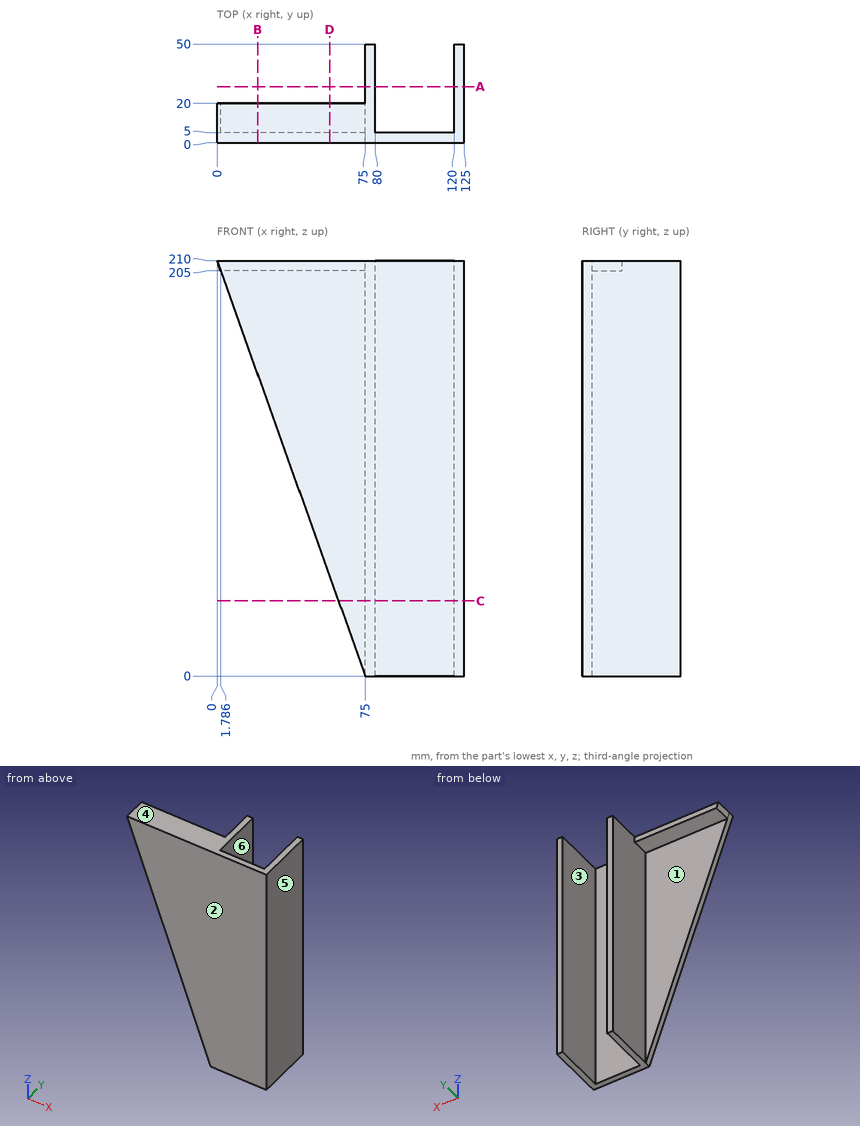
Here's the drawing with two shaded views (mm, measured from the low corner). I have some questions. A direction names the side the tool comes from. Round coordinates to 2 decimals unless told otherwise and drop trailing zeros. Loops run counter-clockwise (first coordinate to the right, second up) from the corner with the lowest first, then second, coordinate; pieces in that order, holes last. Notation, with made-up numbers: (-14.5, 53.5) - (25.5, 53.5) arc R29 ccw to (25.5, 76.5) - close; hole circle Ø8 at (-17, -0.75). An arc over 180 degrees is marked (long way). Write item = value, one per line.
1) Imagine slicing it at A-A (y = 28.5). Please give me the cut outline in (x, z).
Computed:
outline = (75, 0) - (80, 0) - (80, 210) - (75, 210) - close; (120, 0) - (125, 0) - (125, 210) - (120, 210) - close
2) Imagine slicing it at B-B (x = 20.5). Please give me the cut outline in (y, z), and give its area (3 significant figures).
Computed:
outline = (0, 152.6) - (5, 152.6) - (5, 205) - (20, 205) - (20, 210) - (0, 210) - close
area = 362 mm2
3) I'm going to push flat-ended pins straight in: P1, Ø4.5, axis at x = 51, y = 9, coming from the -Z side; P2, Ø4, axis at y = 43.5, z = 97, coming from the -X side; P3, Ø2.5, axis at x = 33.5, z = 207.5, coming from the +Y side. Where does each tip first touch, or does it pass through?
Computed:
P1 = 205
P2 = 75
P3 = 20
4) If we mould it in two halves opening along X, with no side actions, what happens to the marked faces 4, 5 and 6? For each: pulls with the +X half, pulls with the -X half, needs draft (parallel to the pull), parting line crosses it, or undercut.
Computed:
face_4 = needs draft
face_5 = pulls with the +X half
face_6 = undercut
5) Imagine slicing it at D-D (x = 57). Please give me the cut outline in (y, z), and give its area (3 significant figures).
Computed:
outline = (0, 50.4) - (5, 50.4) - (5, 205) - (20, 205) - (20, 210) - (0, 210) - close
area = 873 mm2
6) I need wall thicknesses on line 1 along X through (y, z) = (37.5, 68.5); line 2 along Z through (x, y) = (66.5, 17); line 3 along Y through (x, z) = (103, 177). Which ranges of each line are inside material? Lowest first, please. Write a range as from..to.
Computed:
line_1 = 75..80, 120..125
line_2 = 205..210
line_3 = 0..5
7) On a 3-axis mill with a long thin cutter (end or side, diameter ignored), from which of +Z, -Z, +X, -X, +Y, -Y can I reach the whole of each face in a straight line? I mean the marked faces 1, 2 and 3. Say none if no direction works.
Computed:
face_1 = -Z, -X, +Y
face_2 = +Z, -Z, +X, -X, -Y
face_3 = +Z, -Z, +Y
8) Imagine slicing it at C-C (z = 38). Please give me the cut outline in (x, y).
Computed:
outline = (61.43, 0) - (125, 0) - (125, 50) - (120, 50) - (120, 5) - (80, 5) - (80, 50) - (75, 50) - (75, 5) - (61.43, 5) - close
